Could you check a few things on this model? Use its own coordinates, in mm. A direction names the side the tool comes from. Coordinates: 2 decimals unless noted, no trailing zeros. Write each loop counter-clockwise with the first axis right and the second up, starting at its lowest first coordinate (ties: lowest second). Pieces come first, ordered by that corner, then holes. Notation, with made-up numbers: (8, 21) - (23, 21) arc R24 ccw to (23, 56) - close; hole circle Ø5 at (36, 69.25). An arc over 180 degrees is marked (long way). Answer as a JSON object with one key per item and string values. Group by question number.
1) If we section it at D-D (y = -66.5): Write out the boundary of the cut face in (x, z).
2) If we section it at B-B (z = 18.5): Write out the boundary of the cut face in (x, y).
3) If we section it at C-C (x = 53): Write out the boundary of the cut face in (y, z), plus the area to 3 significant figures.
4) Please list where these lines run through material, in increasing order: line 1 along X through (y, z) = (-12, 28.5); line 2 along Y through (x, z) = (15, 12.5); line 3 along Z through (x, y) = (9, -51).
5) On a 3-axis mill with a long thin cutter (end or side, diameter ignored), from which of +Z, -Z, +X, -X, +Y, -Y can I reach the whole of each face in a straight line? I mean faces 4 (the flat face through (2, -43, 18)), 5 (the flat face through (51, 0, 13)). Say none if no direction works.
6) Will these pins go through, and if not, where does the flat tip stop? pin 1 Ø12 at (x, y) = (24, -60.5) entering from +Z; pin 2 Ø2 at (x, y) = (30.5, -0.5) entering from +Z.
7) We'd pull the mould along Y, two halves only. Please class faces 1 (the flat face through (51, -41, 0)), 2 (the flat face through (102, -43, 18)), 3 (the flat face through (51, -84, 13)): released by +Y, released by -Y, zero draft, split by the parting line, or undercut.
8) If we section it at A-A (y = -34): Write out the boundary of the cut face in (x, z), plus the area to 3 significant figures.
```python
from build123d import *

# Parameters (mm, degrees)
SKETCH006_W     = 104
SKETCH006_H     = 84
SKETCH006_W_2   = 10
SKETCH006_H_2   = 10
PAD002_DEPTH    = 36
SKETCH007_W     = 100
SKETCH007_H     = 80
POCKET004_DEPTH = 34
POCKET005_DEPTH = 84.001
SKETCH009_W     = 90
SKETCH009_H     = 2
POCKET006_DEPTH = 84.001


with BuildPart() as part:
    # Sketch006 (on XY_Plane003 of Origin006) → Pad002 (new body)
    with BuildSketch(Plane.XY):
        with Locations((52, -42)):
            Rectangle(SKETCH006_W, SKETCH006_H)
        with Locations((27.064243, -35)):
            Rectangle(SKETCH006_W_2, SKETCH006_H_2, mode=Mode.SUBTRACT)
    extrude(amount=PAD002_DEPTH)

    # Sketch007 (on Face10 of Pad002) → Pocket004 (cut)
    with BuildSketch(Plane.XY.offset(36)):
        with Locations((52, -42)):
            Rectangle(SKETCH007_W, SKETCH007_H)
    extrude(amount=-POCKET004_DEPTH, mode=Mode.SUBTRACT)

    # Sketch008 (on Face3 of Pocket004) → Pocket005 (cut, through all)
    with BuildSketch(Plane.XZ.offset(84)):
        with BuildLine():
            ThreePointArc((-2.31593, 35.310703), (51.750534, 25.388306), (105.816997, 35.310703))
            Line((105.816997, 35.310703), (106.775558, 49.576915))
            Line((-2.31593, 49.576915), (106.775558, 49.576915))
            Line((-2.31593, 35.310703), (-2.31593, 49.576915))
        make_face()
    extrude(amount=-POCKET005_DEPTH, mode=Mode.SUBTRACT)

    # Sketch009 (on Face5 of Pocket005) → Pocket006 (cut, through all)
    with BuildSketch(Plane(origin=(0, 0, 0), x_dir=(-1, 0, 0), z_dir=(0, 1, 0))):
        with Locations((-52, 21)):
            Rectangle(SKETCH009_W, SKETCH009_H)
    extrude(amount=-POCKET006_DEPTH, mode=Mode.SUBTRACT)


solid = part.part
```
Here are the results:
{
 "1": {"outline": "(0, 0) - (104, 0) - (104, 34.63) arc R152.26 cw to (102, 33.92) - (102, 2) - (2, 2) - (2, 33.75) arc R152.26 cw to (0, 34.45) - close"},
 "2": {"outline": "(0, -84) - (104, -84) - (104, 0) - (0, 0) - close; hole (2, -82) - (102, -82) - (102, -2) - (2, -2) - close"},
 "3": {"outline": "(-84, 0) - (0, 0) - (0, 20) - (-2, 20) - (-2, 2) - (-82, 2) - (-82, 20) - (-84, 20) - close; (-84, 22) - (-82, 22) - (-82, 25.39) - (-84, 25.39) - close; (-2, 22) - (0, 22) - (0, 25.39) - (-2, 25.39) - close", "area": "254 mm²"},
 "4": {"line 1": "x = 0 to 2, 102 to 104", "line 2": "y = -84 to -82, -2 to 0", "line 3": "z = 0 to 2"},
 "5": {"face 4": "+Z", "face 5": "+Z, -Z, +X, -X, +Y"},
 "6": {"pin 1": "stops at z = 2", "pin 2": "stops at z = 27.02"},
 "7": {"face 1": "zero draft", "face 2": "undercut", "face 3": "released by -Y"},
 "8": {"outline": "(0, 0) - (22.06, 0) - (22.06, 2) - (2, 2) - (2, 33.75) arc R152.26 cw to (0, 34.45) - close; (32.06, 0) - (104, 0) - (104, 34.63) arc R152.26 cw to (102, 33.92) - (102, 2) - (32.06, 2) - close", "area": "317 mm²"}
}
